Build history of the part. All positions in model axes, mm. A direction names the side the tool comes from. Coordinates: 2 decimals unless noted, no trailing zeros. Loops run counter-clockwise (first coordinate to the right, second up) from the corner with the lowest first, then second, coordinate; pieces in that order, holes last.
Item 1: Cut at B-B (y = 0). List the corners of the cut face in (x, z), and give its area (3 significant figures).
Item 2: Cut at A-A (z = 0.2). List the corners of the cut face in (x, y), and give its area (3 significant figures).
Item 3: Cut at C-C (x = -4.15). List the corners of the cut face in (y, z).
Item 4: Mould opens along X. For faces 1 (the face through (-7.15, 0, 1)), 2 (the face through (7.15, 0, 1)), 3 (the face through (0.1, -2.5, 1.2)), 4 (the face through (0, 0, 1)) say: released by +X, released by -X, zero draft, split by the parting line, or undercut.
Item 5: 3-axis set-ups, long thin cutter, end or side, ignore diameter. For faces 5 (the face through (1.65, 0, 0.5)), 6 (the face through (0.1, 2.5, 1.2)): which of +Z, -Z, +X, -X, +Y, -Y reach the whole face in a straight line?
Item 6: Flat gauge pin, fed straight in: pin 1 (1.6 mm diameter, centred on x = 0, y = -0.5, fed in from -Z). Where does the tip first touch, or does it go through?
Item 7: Drill centre lines: line 1 along X through (y, z) = (0.75, 1.6); line 2 along X through (y, z) = (1.1, 0.95); line 3 along X through (y, z) = (0.85, 0.95). Where is each one in solid material? Low to high.
Item 8: Cut at D-D (y = 1.65). List the corners of the cut face in (x, z).
from build123d import *

# Parameters (mm, degrees)
SKETCH2_W              = 5
SKETCH2_H              = 14.3
BOSS_EXTRUDE1_DEPTH    = 2
SKETCH2_4_W            = 5
SKETCH2_4_H            = 3.3
CUT_EXTRUDE1_DEPTH     = 1
M2_5_CLEARANCE_HOLE1_D = 2.9


with BuildPart() as part:
    # Sketch2 → Boss-Extrude1 (new body)
    with BuildSketch(Plane(origin=(0, 0, 0), x_dir=(0, 1, 0), z_dir=(0, 0, 1))):
        Rectangle(SKETCH2_W, SKETCH2_H)
    extrude(amount=BOSS_EXTRUDE1_DEPTH)

    # Sketch2<4> → Cut-Extrude1 (cut)
    with BuildSketch(Plane(origin=(0, 0, 0), x_dir=(0, 1, 0), z_dir=(0, 0, 1))):
        Rectangle(SKETCH2_4_W, SKETCH2_4_H)
    extrude(amount=CUT_EXTRUDE1_DEPTH, mode=Mode.SUBTRACT)

    # M2.5 Clearance Hole1 (through all)
    with Locations(Plane.XY.offset(2)):
        with Locations((-4.15, 0), (4.15, 0)):
            Hole(M2_5_CLEARANCE_HOLE1_D / 2)


solid = part.part
Filled sheet:
1. outline: (-7.15, 0) - (-5.6, 0) - (-5.6, 2) - (-7.15, 2) - close; (-2.7, 0) - (-1.65, 0) - (-1.65, 1) - (1.65, 1) - (1.65, 0) - (2.7, 0) - (2.7, 2) - (-2.7, 2) - close; (5.6, 0) - (7.15, 0) - (7.15, 2) - (5.6, 2) - close
1. area: 13.7 mm2
2. outline: (-7.15, -2.5) - (-1.65, -2.5) - (-1.65, 2.5) - (-7.15, 2.5) - close; (1.65, -2.5) - (7.15, -2.5) - (7.15, 2.5) - (1.65, 2.5) - close; hole circle Ø2.9 at (-4.15, 0); hole circle Ø2.9 at (4.15, 0)
2. area: 41.8 mm2
3. outline: (-2.5, 0) - (-1.45, 0) - (-1.45, 2) - (-2.5, 2) - close; (1.45, 0) - (2.5, 0) - (2.5, 2) - (1.45, 2) - close
4. face 1: released by -X
4. face 2: released by +X
4. face 3: zero draft
4. face 4: undercut
5. face 5: -Z, +Y, -Y
5. face 6: +Z, -Z, +X, -X, +Y
6. pin 1: stops at z = 1
7. line 1: x = -7.15 to -5.39, -2.91 to 2.91, 5.39 to 7.15
7. line 2: x = -7.15 to -5.09, -3.21 to -1.65, 1.65 to 3.21, 5.09 to 7.15
7. line 3: x = -7.15 to -5.32, -2.98 to -1.65, 1.65 to 2.98, 5.32 to 7.15
8. outline: (-7.15, 0) - (-1.65, 0) - (-1.65, 1) - (1.65, 1) - (1.65, 0) - (7.15, 0) - (7.15, 2) - (-7.15, 2) - close
